Geometry: see drawing. Coordinates: mm, zero at the bounding-box minimum. A direction names the side the tool comes from. Give positions to 0.01 mm unless a question says otherwise; leave off trailing zeros. Write each loop counter-clockwise with the first axis right and the second up, starting at its lowest first coordinate (ties: lowest second). Pieces come first, ordered by that corner, then holes. Notation, with made-up numbers: M 29,69 L 55,69 A24 cw 55,102 Z; hole C 38.25,23 d1. An arc over 180 degrees is marked long. Use a Markdown table: item, result. Add a question column.
1) Draft query along Y for the marked faces 3, 4 and 5. Return one class per face: +Y half, -Y half, draft (parallel to the pull), parting line (faces both ways), or undercut.
2) Section A-A on y = 13. Return the cut outline in (x, z), then the cut area to 3 significant figures.
3) Set-up query: the marked faces 1 and 2. Return all of +Z, -Z, +X, -X, +Y, -Y with unobstructed straight access to the full face (end or side cutting, diameter ignored); none if empty.
4) Section B-B on x = 3.5. Return the cut outline in (y, z), then the cut area to 3 significant figures.
5) Section C-C on z = 1.1. Return the cut outline in (x, y) (3 decimals), then the cut area to 3 significant figures.
6) Line query: line 1 (Y direction, x = 4.25, z = 2.2); line 2 (X direction, y = 3, z = 1.75); line 3 (Y direction, x = 11.8, z = 2.2) (3 decimals). Output: solid intervals per line, ascending.
7) Section D-D on y = 19.38. Return the cut outline in (x, z) (3 decimals), then the cut area to 3 significant figures.
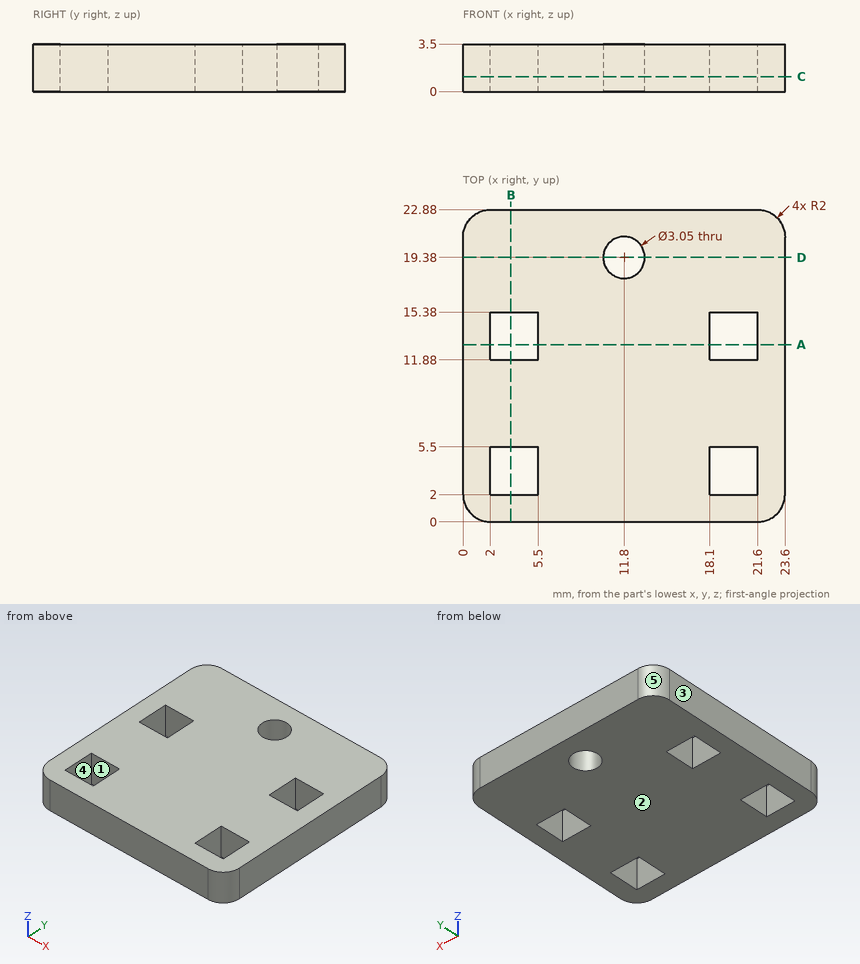
Found:
| question | item | result |
|---|---|---|
| 1 | face 3 | draft |
| 1 | face 4 | undercut |
| 1 | face 5 | +Y half |
| 2 | outline | M 0,0 L 2,0 L 2,3.5 L 0,3.5 Z; M 5.5,0 L 18.1,0 L 18.1,3.5 L 5.5,3.5 Z; M 21.6,0 L 23.6,0 L 23.6,3.5 L 21.6,3.5 Z |
| 2 | area | 58.1 mm² |
| 3 | face 1 | +Z, -Z |
| 3 | face 2 | -Z, +X, -X, +Y, -Y |
| 4 | outline | M 0,0 L 2,0 L 2,3.5 L 0,3.5 Z; M 5.5,0 L 11.88,0 L 11.88,3.5 L 5.5,3.5 Z; M 15.38,0 L 22.88,0 L 22.88,3.5 L 15.38,3.5 Z |
| 4 | area | 55.6 mm² |
| 5 | outline | M 0,2 A2 ccw 2,0 L 21.6,0 A2 ccw 23.6,2 L 23.6,20.88 A2 ccw 21.6,22.88 L 2,22.88 A2 ccw 0,20.88 Z; hole M 2,2 L 5.5,2 L 5.5,5.5 L 2,5.5 Z; hole M 2,11.88 L 5.5,11.88 L 5.5,15.38 L 2,15.38 Z; hole C 11.8,19.38 d3.05; hole M 18.1,2 L 21.6,2 L 21.6,5.5 L 18.1,5.5 Z; hole M 18.1,11.88 L 21.6,11.88 L 21.6,15.38 L 18.1,15.38 Z |
| 5 | area | 480 mm² |
| 6 | line 1 | 0 to 2, 5.5 to 11.88, 15.38 to 22.88 |
| 6 | line 2 | 0 to 2, 5.5 to 18.1, 21.6 to 23.6 |
| 6 | line 3 | 0 to 17.855, 20.905 to 22.88 |
| 7 | outline | M 0,0 L 10.275,0 L 10.275,3.5 L 0,3.5 Z; M 13.325,0 L 23.6,0 L 23.6,3.5 L 13.325,3.5 Z |
| 7 | area | 71.9 mm² |
